Input: part model. Units: mm. Frame: model coordinates. A direction names the side the tool comes from. Coordinates: 2 decimals unless noted, no trailing zeros. Write each loop counter-clockwise with the first axis right and the second up, starting at its lowest first coordinate (ties: lowest second). Pieces come first, ordered by that corner, then holes. Notation, with made-up numbers: (24, -29.5) - (66, -29.5) arc R20 cw to (66, -7.5) - close; hole circle Ø3 at (-17.75, -17). An arc over 180 degrees is marked (long way). Use CSV: the item, a comma, the result in double quotes.
```python
from build123d import *

# Parameters (mm, degrees)
F0_W     = 12.7
F0_H     = 9.525
F0_W_2   = 10.16
F0_H_2   = 6.985
F1_DEPTH = 6.35
F2_R     = 2.54
F3_R     = 2.54
F4_R     = 2.54


with BuildPart() as f1:
    # F0 (on Top) → F1 (new body)
    with BuildSketch(Plane.XY):
        with Locations((6.35, -4.7625)):
            Rectangle(F0_W, F0_H)
        with Locations((6.35, -4.7625)):
            Rectangle(F0_W_2, F0_H_2, mode=Mode.SUBTRACT)
    extrude(amount=F1_DEPTH)

    # F2
    f2_edges = [f1.edges().sort_by_distance(p)[0] for p in [
        (12.7, -9.525, 3.175),
    ]]
    fillet(f2_edges, radius=F2_R)

    # F3
    f3_edges = [f1.edges().sort_by_distance(p)[0] for p in [
        (0, -9.525, 3.175),
    ]]
    fillet(f3_edges, radius=F3_R)

    # F4
    f4_edges = [f1.edges().sort_by_distance(p)[0] for p in [
        (12.7, 0, 3.175),
        (0, 0, 3.175),
    ]]
    fillet(f4_edges, radius=F4_R)


solid = f1.part
```
(1) Cut plane D-D on y = -8.75. Return loops of the section in (x, z), and give its area (3 significant figures).
Check values:
outline,"(0.71, 0) - (11.99, 0) - (11.99, 6.35) - (0.71, 6.35) - close"
area,"71.6 mm^2"
(2) Cut plane B-B on z = 3. Return loops of the section in (x, y) (3 decimals).
Check values:
outline,"(0, -6.985) arc R2.54 ccw to (2.54, -9.525) - (10.16, -9.525) arc R2.54 ccw to (12.7, -6.985) - (12.7, -2.54) arc R2.54 ccw to (10.16, 0) - (2.54, 0) arc R2.54 ccw to (0, -2.54) - close; hole (1.27, -8.255) - (11.43, -8.255) - (11.43, -1.27) - (1.27, -1.27) - close"
(3) Ray query, probe 1 along X at (y, z) = (-3.25, 3); probe 2 along Y at (x, z) = (7.5, 4.5) (3 decimals); probe 3 along X at (y, z) = (-8, 3.75). Return the intervals inside material, ascending. Write a range as from..to.
Check values:
probe 1,"0..1.27, 11.43..12.7"
probe 2,"-9.525..-8.255, -1.27..0"
probe 3,"0.21..1.27, 11.43..12.49"
(4) Draft query along Y for faces 3 (the flat face through (0, -5, 3)), 4 (the flat face through (6, -9.525, 3)), 5 (the cylindrical face through (0.724, -0.764, 3.219)), 6 (the flat face through (11.43, -5, 3)). Return one class per face: pulls with the +Y half, pulls with the -Y half, needs draft (parallel to the pull), parting line crosses it, or undercut.
Check values:
face 3,"needs draft"
face 4,"pulls with the -Y half"
face 5,"pulls with the +Y half"
face 6,"undercut"
(5) Reachability of faces 1 (the flat face through (6, -1.27, 3)), 2 (the flat face through (7, -1, 0)) from +Z, -Z, +X, -X, +Y, -Y: full face, straight path, thin tool, end or side. Return the list, or none.
Check values:
face 1,"+Z, -Z"
face 2,"-Z, +X, -X, +Y, -Y"
(6) Cut plane C-C on y = -5.25. Return loops of the section in (x, z), and give its area (3 significant figures).
Check values:
outline,"(0, 0) - (1.27, 0) - (1.27, 6.35) - (0, 6.35) - close; (11.43, 0) - (12.7, 0) - (12.7, 6.35) - (11.43, 6.35) - close"
area,"16.1 mm^2"
(7) Cut plane A-A on x = 7.5. Return loops of the section in (y, z) (3 decimals).
Check values:
outline,"(-9.525, 0) - (-8.255, 0) - (-8.255, 6.35) - (-9.525, 6.35) - close; (-1.27, 0) - (0, 0) - (0, 6.35) - (-1.27, 6.35) - close"
